CAD build for the part. Positions are in the model's coordinates, mm. Give positions to 0.01 mm unless a question says otherwise; leave off trailing zeros. Order: outer loops, then holes, each group sorted by start corner. A loop starts at its lowest first (then second) coordinate and runs counter-clockwise, first axis right, second up. Notation, with made-up numbers: (-27, 76) -> (9, 76) arc R21 ccw to (9, 88) -> close; hole circle Ø6 at (-11.75, 22). An arc over 180 degrees is marked (long way). Use one line per item in the form item = value. Start each with the question number.
1) Cut at B-B, the plane y = -2. Give the cut face in (x, z) (1 decimal), and give its area (3 significant figures).
2) Probe line 1 (X direction, y = -2.2, z = -0.75); line 2 (X direction, y = -1.15, z = 1); line 3 (Z direction, x = 17.5, y = -1.95). List the from-to ranges inside material, lowest first.
3) Cut at A-A, the plane z = 0. Give the cut face in (x, y).
4) Drop a flat-ended pin along its axis: P1, Ø2.5, axis at x = 17.27, z = 0, coming from the -Y side. Give the stop position or say it passes through.
5) Mould opens along Z. For faces 1 (the face through (21.237, -1.174, -0.087)), 2 (the face through (2, 0, 0)), 3 (the face through (18.844, -0.391, 0.496)) say: pulls with the +Z half, pulls with the -Z half, needs draft (parallel to the pull), parting line crosses it, or undercut.
from build123d import *

# Parameters (mm, degrees)
F0_R     = 1.5875
F0_R_2   = 1.651
F1_DEPTH = 2.38125
F2_SIZE2 = 1.5875
F2_SIZE  = 1.5875


with BuildPart() as f1:
    # F0 (on Front) → F1 (new body)
    with BuildSketch(Plane.XZ):
        with BuildLine():
            Line((17.269202, 3.96875), (-12.893298, 3.96875))
            ThreePointArc((-12.893298, 3.96875), (-16.862048, 0), (-12.893298, -3.96875))
            Line((-12.893298, -3.96875), (17.269202, -3.96875))
            ThreePointArc((17.269202, -3.96875), (21.237952, 0), (17.269202, 3.96875))
        make_face()
        with Locations((-12.893298, 0)):
            Circle(F0_R, mode=Mode.SUBTRACT)
        with Locations((17.269202, 0)):
            Circle(F0_R_2, mode=Mode.SUBTRACT)
    extrude(amount=F1_DEPTH)

    # F2
    f2_edges = [f1.edges().sort_by_distance(p)[0] for p in [
        (15.618202, -2.38125, 0),
    ]]
    chamfer(f2_edges, length=F2_SIZE, length2=F2_SIZE2)


solid = f1.part
Result:
q1.outline = (-12.9, -4) -> (17.3, -4) arc R4 ccw to (17.3, 4) -> (-12.9, 4) arc R4 ccw to start; hole circle Ø3.2 at (-12.9, 0); hole circle Ø5.7 at (17.3, 0)
q1.area = 255 mm²
q2.line_1 = -16.79 to -14.29, -11.49 to 14.31, 20.23 to 21.17
q2.line_2 = -16.73 to -14.13, -11.66 to 15.53, 19.01 to 21.11
q2.line_3 = -3.96 to -2.8, 2.8 to 3.96
q3.outline = (-16.86, -2.38) -> (-14.48, -2.38) -> (-14.48, 0) -> (-16.86, 0) -> close; (-11.31, -2.38) -> (14.03, -2.38) -> (15.62, -0.79) -> (15.62, 0) -> (-11.31, 0) -> close; (18.92, -0.79) -> (20.51, -2.38) -> (21.24, -2.38) -> (21.24, 0) -> (18.92, 0) -> close
q4.P1 = through
q5.face_1 = parting line crosses it
q5.face_2 = needs draft
q5.face_3 = undercut
